The listing builds one solid part. Answer for the finished solid, in the listing's coordinates (mm). Round coordinates to 2 decimals unless told otherwise and drop trailing zeros. Loops run counter-clockwise (first coordinate to the right, second up) from the corner with the lowest first, then second, coordinate; pieces in that order, holes last. Notation, with made-up numbers: (1, 79) - (8, 79) arc R22 ccw to (8, 85) - close; hole circle Ø9 at (-37, -22.75). An arc over 180 degrees is marked (long way). Write item = value, one per line. Start each with the question number.
1) Section C-C, the plane y = -9 is taken. Determine the outline of the cut face in (x, z).
2) Straight lines are drawn through the part: line 1 along Y through (x, z) = (-41.15, -88); line 2 along Z through (x, y) = (-42, -21.5); line 3 along Z through (x, y) = (-43.5, 0). For each, find the intervals that lie inside material, in ascending order.
3) Section B-B, the plane z = 0 is taken. Determine the outline of the cut face in (x, y).
4) Section D-D, the plane z = -33.5 is taken. Determine the outline of the cut face in (x, y), and give its area (4 significant figures).
5) Section A-A, the plane x = -41 is taken. Give the number of separate pieces and of enclosed holes in the cut face, and give its area (3 significant figures).
6) Given pin 1 Ø8 at (y, z) = (-7, 7.5) entering from -X; pin 2 Ø1.5 at (x, z) = (-43.5, -31) entering from -Y; pin 3 Ø4 at (x, y) = (-41.5, 1.5) entering from -Z; pin 4 Ø3.5 at (y, z) = (-15.5, -15.5) entering from +X, each flat-ended and moving along its own axis, determine where each tip first touches the part or whether it passes through.
from build123d import *

# Parameters (mm, degrees)
SKETCH009_R     = 1.5
SKETCH009_R_2   = 13
PAD007_DEPTH    = 5
PAD028_DEPTH    = 6
SKETCH071_W     = 4.5
SKETCH071_H     = 5.5
POCKET019_DEPTH = 2
FILLET002_R     = 1
PAD032_DEPTH    = 5
FILLET003_R     = 5
PAD035_DEPTH    = 5


with BuildPart() as part:
    # Sketch009 (on Face1 of Binder012) → Pad007 (new body)
    with BuildSketch(Plane(origin=(-40, 0, 0), x_dir=(0, -1, 0), z_dir=(-1, 0, 0))):
        with BuildLine():
            Line((-21.15, -17.6144660941), (-21.15, 17.6144660941))
            Line((-21.15, 17.6144660941), (-17.6144660941, 21.15))
            Line((-17.6144660941, 21.15), (17.6144660941, 21.15))
            Line((17.6144660941, 21.15), (21.15, 17.6144660941))
            Line((21.15, 17.6144660941), (21.15, -17.6144660941))
            Line((21.15, -17.6144660941), (21.15, -85))
            Line((21.15, -88), (21.15, -85))
            ThreePointArc((12.15, -88), (16.65, -92.5), (21.15, -88))
            Line((12.15, -85), (12.15, -88))
            Line((-12.15, -85), (12.15, -85))
            Line((-12.15, -88), (-12.15, -85))
            ThreePointArc((-21.15, -88), (-16.65, -92.5), (-12.15, -88))
            Line((-21.15, -85), (-21.15, -88))
            Line((-21.15, -85), (-21.15, -17.6144660941))
        make_face()
        with Locations((-15.5, 15.5)):
            Circle(SKETCH009_R, mode=Mode.SUBTRACT)
        with Locations((15.5, 15.5)):
            Circle(SKETCH009_R, mode=Mode.SUBTRACT)
        with Locations((15.5, -15.5)):
            Circle(SKETCH009_R, mode=Mode.SUBTRACT)
        with Locations((-15.5, -15.5)):
            Circle(SKETCH009_R, mode=Mode.SUBTRACT)
        Circle(SKETCH009_R_2, mode=Mode.SUBTRACT)
        with Locations((-16.65, -88)):
            Circle(SKETCH009_R, mode=Mode.SUBTRACT)
        with Locations((16.65, -88)):
            Circle(SKETCH009_R, mode=Mode.SUBTRACT)
    extrude(amount=PAD007_DEPTH)

    # Sketch070 (on Face23 of Pad007) → Pad028 (join)
    with BuildSketch(Plane(origin=(-45, 0, 0), x_dir=(0, -1, 0), z_dir=(-1, 0, 0))):
        with BuildLine():
            ThreePointArc((12.5199840255, -3.5), (13, 0), (12.5199840255, 3.5))
            Line((12.5199840255, 3.5), (16.5199840255, 3.5))
            Line((16.5199840255, 3.5), (16.5199840255, -3.5))
            Line((16.5199840255, -3.5), (12.5199840255, -3.5))
        make_face()
    extrude(amount=PAD028_DEPTH)

    # Sketch071 (on Face25 of Pad028) → Pocket019 (cut)
    with BuildSketch(Plane.XZ.offset(14.5199840255)):
        with Locations((-47.25, 0.75)):
            Rectangle(SKETCH071_W, SKETCH071_H)
    extrude(amount=-POCKET019_DEPTH, mode=Mode.SUBTRACT)

    # Fillet002
    fillet002_edges = [part.edges().sort_by_distance(p)[0] for p in [
        (-48, -16.519984, 3.5),
        (-48, -16.519984, -3.5),
        (-51, -14.519984, -3.5),
        (-51, -16.519984, 0),
    ]]
    fillet(fillet002_edges, radius=FILLET002_R)

    # Sketch077 (on DatumPlane) → Pad032 (join, symmetric)
    with BuildSketch(Plane(origin=(-44.1666666667, 0, 14.1), x_dir=(-1, 0, 0), z_dir=(0, 1, 0))):
        Polygon((0.8333333333, -27.1), (3.8333333333, -30.1), (3.8333333333, -91.1), (0.8333333333, -94.1), align=None)
    extrude(amount=PAD032_DEPTH, both=True)

    # Fillet003
    fillet003_edges = [part.edges().sort_by_distance(p)[0] for p in [
        (-48, 0, -16),
        (-48, 0, -77),
    ]]
    fillet(fillet003_edges, radius=FILLET003_R)

    # Sketch085 (on Face4 of Fillet003) → Pad035 (join)
    with BuildSketch(Plane(origin=(-45, 0, 0), x_dir=(0, -1, 0), z_dir=(-1, 0, 0))):
        with BuildLine():
            ThreePointArc((21.15, -1.5), (26.15, 3.5), (21.15, 8.5))
            Line((21.15, 10.5), (21.15, 8.5))
            ThreePointArc((21.15, -3.5), (28.15, 3.5), (21.15, 10.5))
            Line((21.15, -1.5), (21.15, -3.5))
        make_face()
    extrude(amount=-PAD035_DEPTH)


solid = part.part
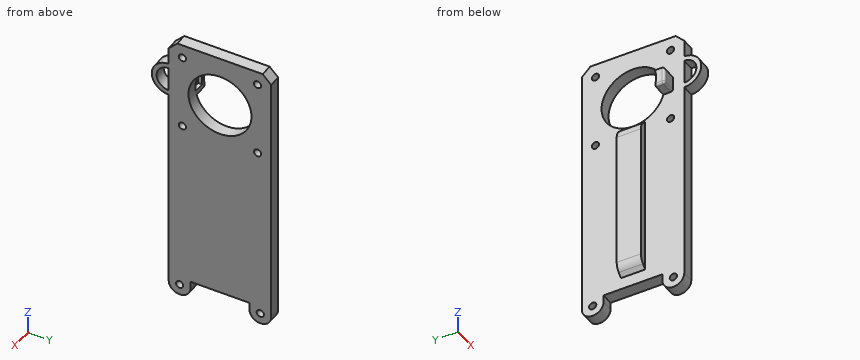
Geometry check:
q1.outline = (-45, -85) - (-40, -85) - (-40, -9.38) - (-45, -9.38) - close; (-45, 9.38) - (-40, 9.38) - (-40, 21.15) - (-45, 21.15) - close
q2.line_1 = -21.15 to -18.15, -15.15 to -12.15, 12.15 to 15.15, 18.15 to 21.15
q2.line_2 = -3.49 to -1.49, 8.49 to 10.49
q2.line_3 = -85 to -13, 13 to 21.15
q3.outline = (-51, -15.52) arc R1 ccw to (-50, -16.52) - (-45, -16.52) - (-45, -21.15) - (-40, -21.15) - (-40, -13) - (-45, -13) - (-45, -14.52) - (-49.5, -14.52) - (-49.5, -13) - (-51, -13) - close; (-45, -27.21) - (-40, -27.21) - (-40, -24.72) - (-45, -24.72) - close; (-45, 13) - (-40, 13) - (-40, 21.15) - (-45, 21.15) - close
q4.outline = (-48, -5) - (-45, -5) - (-45, -21.15) - (-40, -21.15) - (-40, 21.15) - (-45, 21.15) - (-45, 5) - (-48, 5) - close
q4.area = 241.5 mm2
q5.separate_pieces = 1
q5.enclosed_holes = 8
q5.area = 4,060 mm2
q6.pin_1 = -45
q6.pin_2 = -21.15
q6.pin_3 = -85
q6.pin_4 = -40
